Geometry: see drawing. Coordinates: mm, zero at the bounding-box minimum. A direction names the side the tool comes from. Give positions to 0.01 mm unless a question says otherwise; leave off trailing zeros. Write each loop counter-clockwise with the first axis right and the second up, starting at its lowest first coordinate (ties: lowest second). Pieces come first, ordered by that corner, then holes. Notation, with made-up numbers: (52, 36.25) -> (100, 36.25) arc R27 cw to (100, 70.25) -> close; hole circle Ø7 at (-14.75, 65). An arc over 180 degrees is marked (long way). Answer as a JSON object with one key per item and string values. Group by question number.
Item 1: Section query B-B on y = 60. Return the cut outline in (x, z), plus the area to 3 significant figures.
Item 2: First-contact query: pin 1 Ø6 at (y, z) = (34, 69) entering from -X; pin 2 Ø12 at (y, z) = (27.5, 65) entering from +X. Flat tips, straight axial feed; report the tip coordinate or a pass-through.
Item 3: Section query C-C on x = 75. Return the cut outline in (y, z), plus the area to 3 significant figures.
Item 4: Section query A-A on z = 69. Return the cut outline in (x, y).
Item 5: Section query D-D on z = 46.5. Return the cut outline in (x, y).
Item 6: Access query for the marked faces 1 and 2. Directions: +Z, -Z, +X, -X, +Y, -Y. A direction counts if a zero-diameter tool reaches every point of the face in a straight line with its end or side. Return the directions, or none.
Item 7: Pull-direction query (X, two-part tool) for the marked faces 3, 4, 5 and 6; classes: pulls with the +X half, pulls with the -X half, needs draft (parallel to the pull), parting line crosses it, or undercut.
Item 8: Ray query, probe 1 along Z at (x, y) = (324, 49); probe 2 along Z at (x, y) = (190.5, 72); probe 3 along X at (y, z) = (86.5, 65) (1 decimal). Return the intervals inside material, ascending. Write a range as from..to.
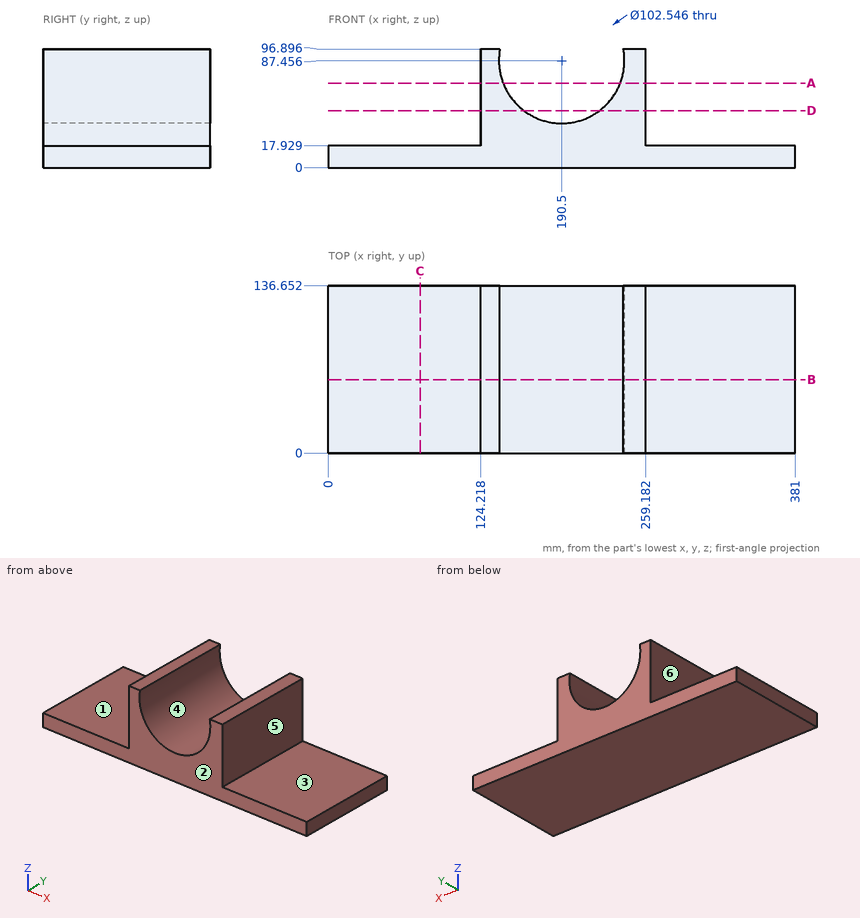
Worked answers:
{
 "1": {"outline": "(0, 0) -> (381, 0) -> (381, 17.93) -> (259.18, 17.93) -> (259.18, 96.9) -> (240.9, 96.9) arc R51.27 cw (long way) to (140.1, 96.9) -> (124.22, 96.9) -> (124.22, 17.93) -> (0, 17.93) -> close", "area": "12,400 mm^2"},
 "2": {"pin 1": "x = 124.22", "pin 2": "x = 259.18"},
 "3": {"outline": "(0, 0) -> (136.65, 0) -> (136.65, 17.93) -> (0, 17.93) -> close", "area": "2,450 mm^2"},
 "4": {"outline": "(124.22, 0) -> (142.66, 0) -> (142.66, 136.65) -> (124.22, 136.65) -> close; (238.34, 0) -> (259.18, 0) -> (259.18, 136.65) -> (238.34, 136.65) -> close"},
 "5": {"outline": "(124.22, 0) -> (159.65, 0) -> (159.65, 136.65) -> (124.22, 136.65) -> close; (221.35, 0) -> (259.18, 0) -> (259.18, 136.65) -> (221.35, 136.65) -> close"},
 "6": {"face 1": "+Z, -X, +Y, -Y", "face 2": "+Z, -Z, +X, -X, -Y"},
 "7": {"face 3": "needs draft", "face 4": "undercut", "face 5": "pulls with the +X half", "face 6": "pulls with the -X half"},
 "8": {"probe 1": "0..17.93", "probe 2": "0..36.18", "probe 3": "124.2..144.4, 236.6..259.2"}
}
